from build123d import *

# Parameters (mm, degrees)
BOSS_EXTRUDE1_DEPTH      = 15
BOSS_EXTRUDE2_DEPTH      = 55
BOSS_EXTRUDE2_DEPTH_BACK = 15
SKETCH2_R                = 30
HOLE1_D                  = 46
SKETCH5_W                = 50
SKETCH5_H                = 55
BOSS_EXTRUDE3_DEPTH      = 15
RIB1_REACH               = 133.743
SKETCH6_WALL_W           = 300.486242526
SKETCH6_WALL_H           = 6
BOSS_EXTRUDE5_DEPTH      = 3
HOLE2_D                  = 25


with BuildPart() as part:
    # Sketch1 → Boss-Extrude1 (new body)
    with BuildSketch(Plane(origin=(0, 0, 0), x_dir=(0, 0, -1), z_dir=(1, 0, 0))):
        with BuildLine():
            Line((-80, 27.5), (80, 27.5))
            Line((80, 27.5), (80, -27.5))
            Line((80, -27.5), (-80, -27.5))
            ThreePointArc((-80, -27.5), (-107.5, 0), (-80, 27.5))
        make_face()
    extrude(amount=BOSS_EXTRUDE1_DEPTH)

    # Sketch2 → Boss-Extrude2 (add, two sides: drawn at the far end of the back side and taken through both)
    with BuildSketch(Plane(origin=(15, 0, 0), x_dir=(0, 0, -1), z_dir=(1, 0, 0)).offset(-BOSS_EXTRUDE2_DEPTH_BACK)):
        Circle(SKETCH2_R)
    extrude(amount=BOSS_EXTRUDE2_DEPTH + BOSS_EXTRUDE2_DEPTH_BACK)

    # Hole1 (through all)
    with Locations(Plane(origin=(70, 0, 0), x_dir=(0, 0, -1), z_dir=(1, 0, 0))):
        with Locations((0, 0)):
            Hole(HOLE1_D / 2)

    # Sketch5 → Boss-Extrude3 (add)
    with BuildSketch(Plane(origin=(0, 0, -80), x_dir=(-1, 0, 0), z_dir=(0, 0, -1))):
        with Locations((-25, 0)):
            Rectangle(SKETCH5_W, SKETCH5_H)
    extrude(amount=-BOSS_EXTRUDE3_DEPTH)

    # Sketch6 wall → Rib1 (add, up to next)
    with BuildSketch(Plane(origin=(50, 0, -47.5), x_dir=(0, 0, 1), z_dir=(1, 0, 0)), mode=Mode.PRIVATE) as rib1_sk1:
        Rectangle(SKETCH6_WALL_W, SKETCH6_WALL_H)
    rib1_tool1 = extrude(rib1_sk1.sketch, amount=-RIB1_REACH, mode=Mode.PRIVATE) - part.part
    add(rib1_tool1.solids().sort_by_distance((50, 0, -47.5))[0])

    # Sketch7 → Boss-Extrude5 (add, symmetric)
    with BuildSketch(Plane(origin=(0, 0, 0), x_dir=(1, 0, 0), z_dir=(0, 1, 0))):
        Polygon((70, -30), (15, -55), (15, -28), (70, -28), align=None)
    extrude(amount=BOSS_EXTRUDE5_DEPTH, both=True)

    # Hole2 (through all)
    with Locations(Plane(origin=(15, 0, 0), x_dir=(0, 0, -1), z_dir=(1, 0, 0))):
        with Locations((-80, 0)):
            Hole(HOLE2_D / 2)


solid = part.part
Model file for the job. Use its own axes, mm. A direction names the side the tool comes from. Give positions to 0.01 mm unless a question says otherwise; leave off trailing zeros. Order: outer loops, then holes, each group sorted by start corner. A loop starts at its lowest first (then second) coordinate and runs counter-clockwise, first axis right, second up. Notation, with made-up numbers: (-2, 20) - (38, 20) arc R26 ccw to (38, 45) - close; hole circle Ø3 at (-4, 30.5). An arc over 180 degrees is marked (long way). Write item = value, one per line. Start each with the question number.
1. Which spindle directions (+Z, -Z, +X, -X, +Y, -Y) get a long thin tool onto all of the face, cutting with end or side? Do faces 4 (the flat face through (50, 0, -66)), 5 (the flat face through (37, 3, 39)), 6 (the flat face through (33, 3, -48)), 7 (the flat face through (7, 27.5, 46)). Say none if no direction does.
2. Cut at A-A, the plane y = 0. List the corners of the cut face in (x, z).
3. Drop flat-ended pins along their axis: P1, Ø6, axis at y = -7, z = 81, coming from the -X side; P2, Ø19.5, axis at x = 32, y = 20, coming from the +Z side; P3, Ø6, axis at x = 23, y = -17, coming from the +Z side; P4, Ø1.5, axis at x = 10, z = 68, coming from the -Y side. Give the stop position or say it passes through.
4. Cut at C-C, the plane x = 28. List the corners of the cut face in (y, z).
5. Cut at D-D, the plane y = 17.5. List the corners of the cut face in (x, z).
6. Cut at B-B, the plane z = 70. List the corners of the cut face in (x, y), and give its area (3 significant figures).
7. Probe line 1 along Z through (x, y) = (47.5, 21); line 2 along X through (y, z) = (13, -40); line 3 along X through (y, z) = (15, -70). List the from-to ranges inside material, lowest first.
8. Two-plate mould, pull along Y, no slides. Class faces 1 (the cylindrical face through (42.29, 13.87, 26.6)), 2 (the flat face through (33, 15, -65)), 3 (the cylindrical face through (34.51, 22.804, -2.994)): pulls with the +Y half, pulls with the -Y half, needs draft (parallel to the pull), parting line crosses it, or undercut.
Taken from the geometry:
q1.face_4 = -Z, +X, +Y, -Y
q1.face_5 = +Z, +X, +Y
q1.face_6 = +X, +Y
q1.face_7 = +Z, +X, -X, +Y
q2.outline = (0, -80) - (50, -80) - (50, -30) - (70, -30) - (70, -23) - (0, -23) - close; (0, 23) - (70, 23) - (70, 30) - (15, 55) - (15, 67.5) - (0, 67.5) - close; (0, 92.5) - (15, 92.5) - (15, 107.5) - (0, 107.5) - close
q3.P1 = through
q3.P2 = 28.19
q3.P3 = 26.53
q3.P4 = -27.5
q4.outline = (-27.5, -80) - (27.5, -80) - (27.5, -65) - (3, -65) - (3, -29.85) arc R30 ccw to (3, 29.85) - (3, 49.09) - (-3, 49.09) - (-3, 29.85) arc R30 ccw to (-3, -29.85) - (-3, -65) - (-27.5, -65) - close; hole circle Ø46 at (0, 0)
q5.outline = (0, -80) - (50, -80) - (50, -65) - (15, -65) - (15, -24.37) - (70, -24.37) - (70, -14.92) - (0, -14.92) - close; (0, 14.92) - (70, 14.92) - (70, 24.37) - (15, 24.37) - (15, 101.21) - (0, 101.21) - close
q6.outline = (0, -27.5) - (15, -27.5) - (15, -7.5) - (0, -7.5) - close; (0, 7.5) - (15, 7.5) - (15, 27.5) - (0, 27.5) - close
q6.area = 600 mm²
q7.line_1 = -80 to -65, -21.42 to -9.38, 9.38 to 21.42
q7.line_2 = 0 to 15
q7.line_3 = 0 to 50
q8.face_1 = parting line crosses it
q8.face_2 = needs draft
q8.face_3 = undercut
